Could you check a few things on this model? Use its own coordinates, in mm. A direction names the side the tool comes from. Round coordinates to 2 decimals unless told otherwise and drop trailing zeros. Write each loop counter-clockwise with the first axis right and the second up, starting at its lowest first coordinate (ties: lowest second). Pieces come first, ordered by that corner, then holes. Notation, with made-up numbers: (68, 66.25) -> (91, 66.25) arc R32 ccw to (91, 92.25) -> close; hole circle Ø8 at (76.25, 17.5). An arc over 180 degrees is marked (long way). One line per question, with ' | ' between items. Start each with the question number.
1. For pin 1 Ø7 at (x, y) = (-9, 0.5) entering from +Z; pin 2 Ø3 at (y, z) = (-2.5, 9) entering from -X; pin 3 Ø10 at (y, z) = (7, 13) entering from -X, each with a flat end and sliding along its axis, tell me the tip position at first contact or that it passes through.
2. Thinking about a two-plate mould opening in X: for faces 1 (the flat face through (-8, 9.5, 8)), 2 (the flat face through (16.02, 6.93, 6.87)), 3 (the cylindrical face through (-20.3, 0, 8.9)), 4 (the flat face through (9, 0, 0)), which applies, released by +X, released by -X, zero draft, split by the parting line, or undercut?
3. Imagine slicing it at C-C, the plane z = 1.5. List the corners of the cut face in (x, y) for me, and give its area (3 significant figures).
4. Imagine slicing it at B-B, the plane x = 0. List the corners of the cut face in (y, z) for me.
5. If I drill on line 1 along Y through (x, z) = (0, 12); line 2 along Y through (x, z) = (9, 6.5); line 3 along Z through (x, y) = (-11.5, 9), over which ranges is the centre line in solid material (lowest first)? Write a range as [from, to].
6. Imagine slicing it at A-A, the plane y = 0. List the corners of the cut face in (x, z) for me, and give its area (3 significant figures).
7. For faces 5 (the cylindrical face through (15.14, -5.92, 15.54)), 6 (the flat face through (10, 0, 2.5)), 7 (the cylindrical face through (-15.14, 5.92, 15.54)), which set-ups out of +Z, -Z, +X, -X, +Y, -Y let a thin tool reach every point of the face, with its end or its side?
8. Imagine slicing it at D-D, the plane y = -8. List the corners of the cut face in (x, z) for me, and give its area (3 significant figures).
from build123d import *

# Parameters (mm, degrees)
SKETCH_R        = 1.6
PAD_DEPTH       = 2.5
SKETCH001_R     = 1.6
SKETCH001_W     = 24.2
SKETCH001_H     = 19
PAD001_DEPTH    = 15.5
SKETCH002_W     = 27.5
SKETCH002_H     = 25
POCKET_DEPTH    = 5
POCKET001_DEPTH = 18.001
FILLET_R        = 2


with BuildPart() as part:
    # Sketch → Pad (new body)
    with BuildSketch(Plane.XY):
        with BuildLine():
            Line((-12.1, 12), (12.1, 12))
            Line((12.1, 12), (19.442827, 2.508799))
            ThreePointArc((19.442837, -2.508786), (20.3, 8e-06), (19.442827, 2.508799))
            Line((19.442837, -2.508786), (12.1, -12))
            Line((12.1, -12), (-12.1, -12))
            Line((-12.1, -12), (-19.442827, -2.508799))
            ThreePointArc((-19.442827, 2.508799), (-20.3, 0), (-19.442827, -2.508799))
            Line((-12.1, 12), (-19.442827, 2.508799))
        make_face()
        with Locations((-16.2, 0)):
            Circle(SKETCH_R, mode=Mode.SUBTRACT)
        with Locations((16.2, 0)):
            Circle(SKETCH_R, mode=Mode.SUBTRACT)
    extrude(amount=PAD_DEPTH)

    # Sketch001 (on Face12 of Pad) → Pad001 (join)
    with BuildSketch(Plane.XY.offset(2.5)):
        with BuildLine():
            Line((-12.1, 12), (-19.442827, 2.508799))
            ThreePointArc((-19.442827, 2.508799), (-20.3, 0), (-19.442827, -2.508799))
            Line((-12.1, -12), (-19.442827, -2.508799))
            Line((12.1, -12), (-12.1, -12))
            Line((19.442837, -2.508786), (12.1, -12))
            ThreePointArc((19.442837, -2.508786), (20.3, 8e-06), (19.442827, 2.508799))
            Line((12.1, 12), (19.442827, 2.508799))
            Line((-12.1, 12), (12.1, 12))
        make_face()
        with Locations((-16.2, 0)):
            Circle(SKETCH001_R, mode=Mode.SUBTRACT)
        with Locations((16.2, 0)):
            Circle(SKETCH001_R, mode=Mode.SUBTRACT)
        Rectangle(SKETCH001_W, SKETCH001_H, mode=Mode.SUBTRACT)
    extrude(amount=PAD001_DEPTH)

    # Sketch002 (on Face15 of Pad001) → Pocket (cut)
    with BuildSketch(Plane.XY.offset(18)):
        Rectangle(SKETCH002_W, SKETCH002_H)
    extrude(amount=-POCKET_DEPTH, mode=Mode.SUBTRACT)

    # Sketch003 (on Face4 of Pocket) → Pocket001 (cut, through all)
    with BuildSketch(Plane(origin=(0, 0, 0), x_dir=(1, 0, 0), z_dir=(0, 0, -1))):
        with BuildLine():
            ThreePointArc((8, 2.3), (0, 10.3), (-8, 2.3))
            Line((-8, 2.3), (-8, -2.3))
            ThreePointArc((-8, -2.3), (0, -10.3), (8, -2.3))
            Line((8, -2.3), (8, 2.3))
        make_face()
    extrude(amount=-POCKET001_DEPTH, mode=Mode.SUBTRACT)

    # Fillet
    fillet_edges = [part.edges().sort_by_distance(p)[0] for p in [
        (-12.1, 12, 7.75),
        (12.1, 12, 7.75),
        (12.1, -12, 7.75),
        (-12.1, -12, 7.75),
        (-13.75, -9.867241, 15.5),
        (13.75, -9.867241, 15.5),
        (13.75, 9.867241, 15.5),
        (-13.75, 9.867241, 15.5),
    ]]
    fillet(fillet_edges, radius=FILLET_R)


solid = part.part
Geometry results:
1) pin 1: stops at z = 13 | pin 2: stops at x = -20.18 | pin 3: stops at x = -19.78
2) face 1: undercut | face 2: released by +X | face 3: released by -X | face 4: zero draft
3) outline: (-19.44, -2.51) -> (-12.7, -11.22) arc R2 ccw to (-11.12, -12) -> (11.12, -12) arc R2 ccw to (12.7, -11.22) -> (19.44, -2.51) arc R4.1 ccw to (19.44, 2.51) -> (12.7, 11.22) arc R2 ccw to (11.12, 12) -> (-11.12, 12) arc R2 ccw to (-12.7, 11.22) -> (-19.44, 2.51) arc R4.1 ccw to start; hole circle Ø3.2 at (-16.2, 0); hole (-8, -2.3) arc R8 ccw to (8, -2.3) -> (8, 2.3) arc R8 ccw to (-8, 2.3) -> close; hole circle Ø3.2 at (16.2, 0) | area: 508 mm2
4) outline: (-12, 0) -> (-10.3, 0) -> (-10.3, 13) -> (-12, 13) -> close; (10.3, 0) -> (12, 0) -> (12, 13) -> (10.3, 13) -> close
5) line 1: y = [-12, -10.3], [10.3, 12] | line 2: y = [-12, -9.5], [9.5, 12] | line 3: z = [0, 2.5]
6) outline: (-20.3, 0) -> (-17.8, 0) -> (-17.8, 18) -> (-20.3, 18) -> close; (-14.6, 0) -> (-8, 0) -> (-8, 2.5) -> (-12.1, 2.5) -> (-12.1, 13) -> (-13.75, 13) -> (-13.75, 18) -> (-14.6, 18) -> close; (8, 0) -> (14.6, 0) -> (14.6, 18) -> (13.75, 18) -> (13.75, 13) -> (12.1, 13) -> (12.1, 2.5) -> (8, 2.5) -> close; (17.8, 0) -> (20.3, 0) -> (20.3, 18) -> (17.8, 18) -> close | area: 184 mm2
7) face 5: +Z, -Y | face 6: +Z | face 7: +Z, +Y
8) outline: (-15.19, 0) -> (-5.61, 0) -> (-5.61, 2.5) -> (-12.1, 2.5) -> (-12.1, 13) -> (-15.19, 13) -> close; (5.61, 0) -> (15.19, 0) -> (15.19, 13) -> (12.1, 13) -> (12.1, 2.5) -> (5.61, 2.5) -> close | area: 113 mm2
